Verification items for this drawing (mm, ordinates from the low corner). A direction names the side the tool comes from. Round coordinates to 2 decimals unless told otherwise and drop trailing zeros. Order: outer loops, then holes, each group sorted by start corner. A loop starts at its lowest first (then second) coordinate and runs counter-clockwise, first axis right, second up. Notation, with made-up numbers: (35, -1.5) -> (40, -1.5) arc R28 cw to (40, 17.5) -> close; hole circle Ø4 at (17, -10). An arc over 180 degrees is marked (long way). Put each result on its own line as item: value.
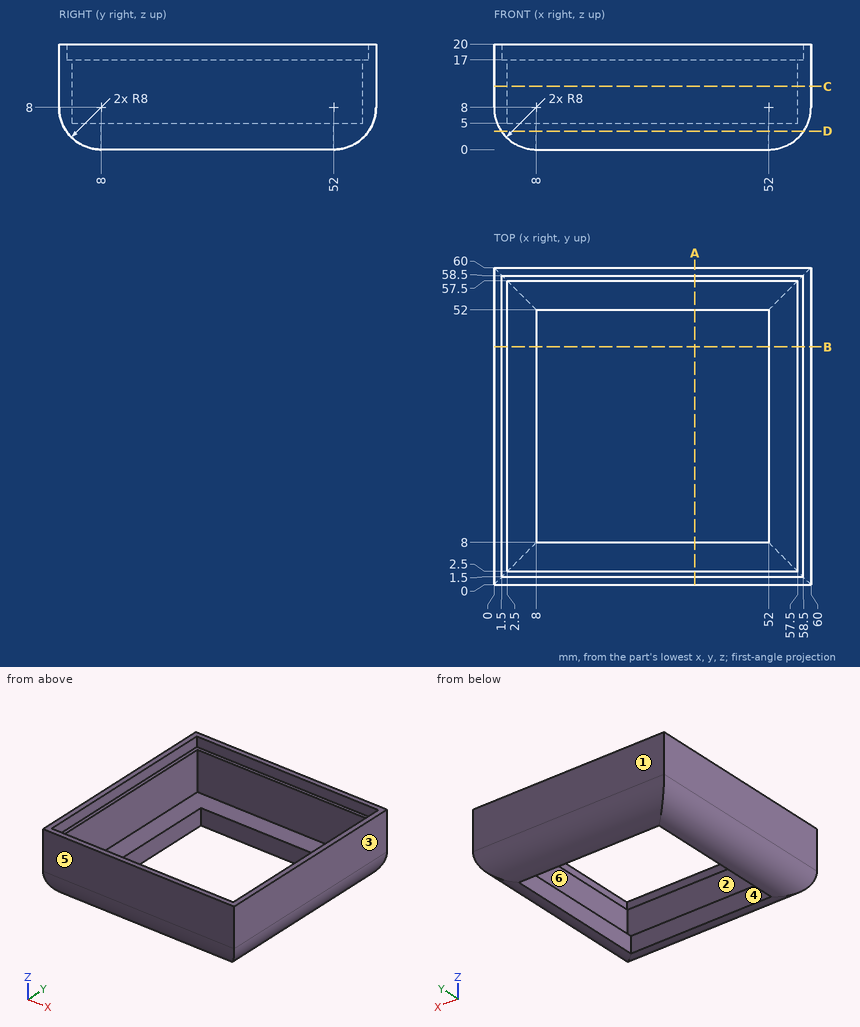
Item 1: Release check for a two-part mould opening along X. For the marked faces 1, 2 and 3 record: +X half, -X half, draft (parallel to the pull), parting line (faces both ways), or undercut.
Check sheet entries:
face 1: draft
face 2: undercut
face 3: +X half
Item 2: Material ranges on L1, parallel to Y at x = 29, z = 8.5; L2, parallel to Y at x = 3, z = 18.5, recorded low to high. Write a range as [from, to].
Check sheet entries:
L1: y = [0, 2.5], [57.5, 60]
L2: y = [0, 1.5], [58.5, 60]
Item 3: Section check A-A on x = 38. Record the boundary of the cut face in (y, z), then the cut area to 3 significant figures.
Check sheet entries:
outline: (0, 8) arc R8 ccw to (8, 0) -> (8, 5) -> (2.5, 5) -> (2.5, 17) -> (1.5, 17) -> (1.5, 20) -> (0, 20) -> close; (52, 0) arc R8 ccw to (60, 8) -> (60, 20) -> (58.5, 20) -> (58.5, 17) -> (57.5, 17) -> (57.5, 5) -> (52, 5) -> close
area: 122 mm^2
Item 4: Gauge pin test, flat ends, axial feed: pin 1 Ø3 at (y, z) = (9.5, 6.5) entering from -X; pin 2 Ø2 at (y, z) = (39, 5) entering from -X; pin 3 Ø5.5 at (x, z) = (27, 3) entering from +Y; pin 4 Ø2 at (x, z) = (51, 2.5) entering from -Y. Record the tip position at first contact, or that the pin passes through.
Check sheet entries:
pin 1: stops at x = 0
pin 2: stops at x = 0.25
pin 3: stops at y = 59.68
pin 4: stops at y = 1.39
Item 5: Section check C-C on z = 12. Record the boundary of the cut face in (x, y), then the cut area to 3 significant figures.
Check sheet entries:
outline: (0, 0) -> (60, 0) -> (60, 60) -> (0, 60) -> close; hole (2.5, 2.5) -> (57.5, 2.5) -> (57.5, 57.5) -> (2.5, 57.5) -> close
area: 575 mm^2
Item 6: Section check D-D on z = 3.5. Record the boundary of the cut face in (x, y).
Check sheet entries:
outline: (1.39, 1.39) -> (58.61, 1.39) -> (58.61, 58.61) -> (1.39, 58.61) -> close; hole (8, 8) -> (52, 8) -> (52, 52) -> (8, 52) -> close
Item 7: Tool access check on the marked faces 4, 5 and 6. Record the directions out of +Z, -Z, +X, -X, +Y, -Y that give a thin tool (end or side, any length) a straight path to the whole face; none if there is none.
Check sheet entries:
face 4: +Z, -Z
face 5: +Z, -Z, +X, -X, -Y
face 6: +Z
